Part model, mm, in its own coordinate system. A direction names the side the tool comes from. Coordinates: 2 decimals unless noted, no trailing zeros. Order: outer loops, then holes, each group sorted by start corner. A loop starts at its lowest first (then second) coordinate and runs counter-clockwise, first axis right, second up.
```python
from build123d import *

# Parameters (mm, degrees)
SKETCH1_W           = 50
SKETCH1_H           = 41
BOSS_EXTRUDE1_DEPTH = 5
SKETCH2_W           = 15
SKETCH2_H           = 15
BOSS_EXTRUDE2_DEPTH = 50
BOSS_EXTRUDE3_DEPTH = 5
FILLET1_START       = -20.5
FILLET1_DEPTH       = 41
FILLET1_2_DEPTH     = 15
FILLET2_R           = 10


with BuildPart() as part:
    # Sketch1 → Boss-Extrude1 (new body)
    with BuildSketch(Plane(origin=(0, 0, 0), x_dir=(0, 0, -1), z_dir=(1, 0, 0))):
        Rectangle(SKETCH1_W, SKETCH1_H)
    extrude(amount=BOSS_EXTRUDE1_DEPTH)

    # Sketch2 → Boss-Extrude2 (add)
    with BuildSketch(Plane.ZY):
        with Locations((0, -13)):
            Rectangle(SKETCH2_W, SKETCH2_H)
    extrude(amount=BOSS_EXTRUDE2_DEPTH)

    # Sketch3 → Boss-Extrude3 (add)
    with BuildSketch(Plane(origin=(5, 0, 0), x_dir=(0, 0, -1), z_dir=(1, 0, 0))):
        with BuildLine():
            Line((25, 20.5), (-25, 20.5))
            Line((-25, 20.5), (-25, -0.4))
            Line((-25, -0.4), (-20.1, -0.4))
            ThreePointArc((-20.1, -0.4), (0, 19.7), (20.1, -0.4))
            Line((20.1, -0.4), (20.1, -20.5))
            Line((20.1, -20.5), (25, -20.5))
            Line((25, -20.5), (25, 20.5))
        make_face()
    extrude(amount=BOSS_EXTRUDE3_DEPTH)

    # Fillet1: read off the stored shape, not the designer's step
    # Fillet1 outline → Fillet1 (cut)
    with BuildSketch(Plane(origin=(0, 0, 0), x_dir=(1, 0, 0), z_dir=(0, 1, 0)).offset(FILLET1_START)):
        with BuildLine():
            Line((-50, 7.5), (-50, 0))
            ThreePointArc((-50, 0), (-47.803300859, 5.303300859), (-42.5, 7.5))
            Line((-42.5, 7.5), (-50, 7.5))
        make_face()
        with BuildLine():
            ThreePointArc((-42.5, -7.5), (-47.803300859, -5.303300859), (-50, 0))
            Line((-50, 0), (-50, -7.5))
            Line((-50, -7.5), (-42.5, -7.5))
        make_face()
    extrude(amount=FILLET1_DEPTH, mode=Mode.SUBTRACT)

    # Fillet1 2 outline → Fillet1 2 (add)
    with BuildSketch(Plane(origin=(0, 0, 0), x_dir=(1, 0, 0), z_dir=(0, 1, 0)).offset(FILLET1_START)):
        with BuildLine():
            Line((0, -7.5), (-7.5, -7.5))
            ThreePointArc((-7.5, -7.5), (-2.196699141, -9.696699141), (0, -15))
            Line((0, -15), (0, -7.5))
        make_face()
        with BuildLine():
            ThreePointArc((0, 15), (-2.196699141, 9.696699141), (-7.5, 7.5))
            Line((-7.5, 7.5), (0, 7.5))
            Line((0, 7.5), (0, 15))
        make_face()
    extrude(amount=FILLET1_2_DEPTH)

    # Fillet2
    fillet2_edges = [part.edges().sort_by_distance(p)[0] for p in [
        (5, 20.5, 25),
        (5, 20.5, -25),
    ]]
    fillet(fillet2_edges, radius=FILLET2_R)


solid = part.part
```
(1) Probe line 1 (X direction, y = 0, z = -7); line 2 (X direction, y = -7.5, z = -22); line 3 (Z direction, x = -20, y = -13). List the from-to ranges inside material, lowest first.
(2) Drop flat-ended pins along their axis: pin 1 (4.5 mm diameter, centred on x = -27, y = -12, fed in from +Z); pin 2 (20.5 mm diameter, centred on y = 9.5, z = 9, fed in from -X); pin 3 (7.5 mm diameter, centred on x = -24.5, y = -14.5, fed in from -Z); pin 4 (3 mm diameter, centred on x = -1.5, z = -11, fed in from -Y). Give the stop position or say it passes through.
(3) Pull direction Z, two halves, no side cores. Call faces 1 (the face through (4, -1, 25)), 2 (the face through (4.93, 17.49, -22.15)), 3 (the face through (7.465, 19.695, 0.442)): +Z half, -Z half, draft (parallel to the pull), parting line (faces both ways), or undercut.
(4) Slice it at B-B, the plane x = 6. Give the cut face in (y, z).
(5) Slice it at C-C, the plane z = 14. Give the cut face in (x, y).
(6) Slice it at A-A, the plane y = -8. Give the cut face in (x, z), then the cut area to 3 significant figures.
(7) Tool access for faces 4 (the face through (5, 0, 3)), 5 (the face through (-25, -13, -7.5)), 6 (the face through (-25, -5.5, 0)), 7 (the face through (7, -0.4, 23)): list every direction of +Z, -Z, +X, -X, +Y, -Y with a clear straight run to the whole face (end or side of a thin tool).
(8) Slice it at D-D, the plane x = -24. Give the cut face in (y, z).
Here are the results:
1. line 1: x = 0 to 5
1. line 2: x = 0 to 10
1. line 3: z = -7.5 to 7.5
2. pin 1: stops at z = 7.5
2. pin 2: stops at x = 0
2. pin 3: stops at z = -7.5
2. pin 4: stops at y = -20.5
3. face 1: +Z half
3. face 2: -Z half
3. face 3: undercut
4. outline: (-20.5, -25) - (10.5, -25) arc R10 ccw to (20.5, -15) - (20.5, 15) arc R10 ccw to (10.5, 25) - (-0.4, 25) - (-0.4, 20.1) arc R20.1 cw to (-0.4, -20.1) - (-20.5, -20.1) - close
5. outline: (-0.07, -20.5) - (5, -20.5) - (5, 14.02) - (10, 14.02) - (10, 20.5) - (0, 20.5) - (0, -5.5) - (-0.07, -5.5) - close
6. outline: (-42.5, -7.5) - (-7.5, -7.5) arc R7.5 cw to (0, -15) - (0, -25) - (10, -25) - (10, -20.1) - (5, -20.1) - (5, 25) - (0, 25) - (0, 15) arc R7.5 cw to (-7.5, 7.5) - (-42.5, 7.5) arc R7.5 ccw to start
6. area: 1,020 mm2
7. face 4: +X, -Y
7. face 5: -Z, -X, +Y, -Y
7. face 6: +Z, -Z, -X, +Y
7. face 7: +Z, +X, -Y
8. outline: (-20.5, -7.5) - (-5.5, -7.5) - (-5.5, 7.5) - (-20.5, 7.5) - close
